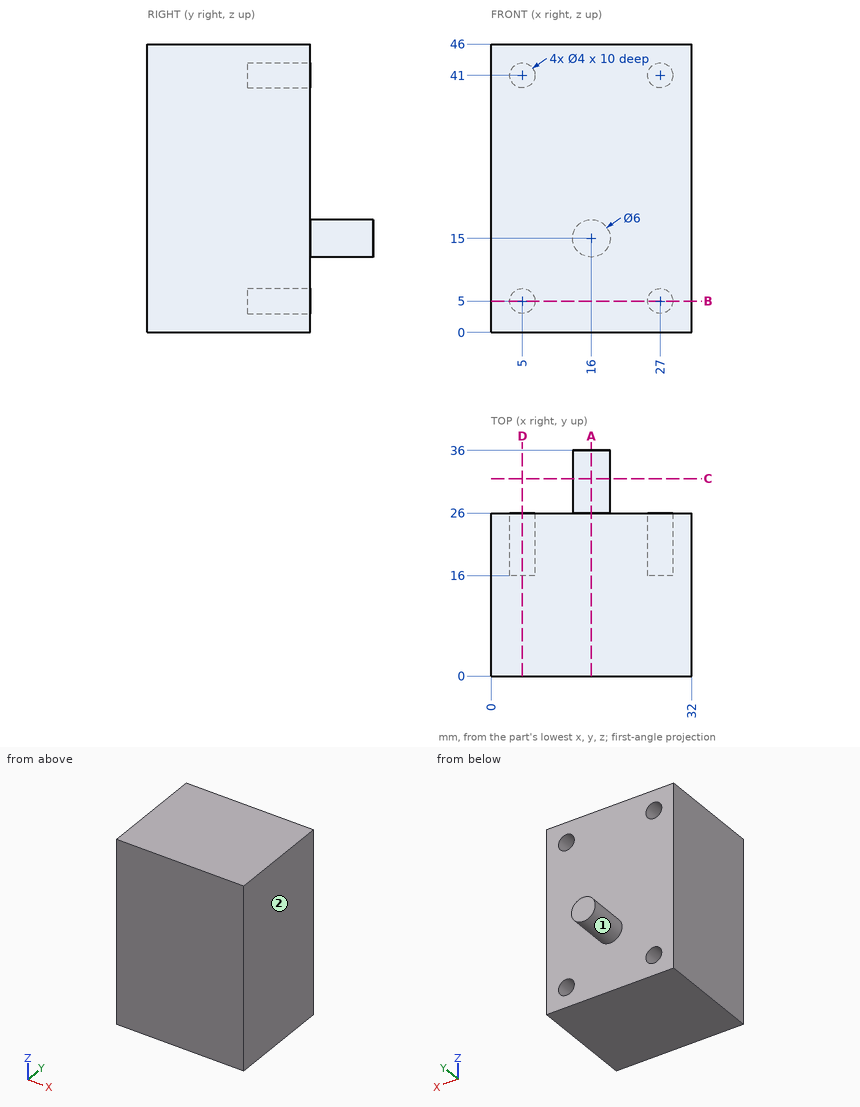
Could you check a few things on this drawing? It's one solid part, dimensions in mm from its lowest x, y, z. A direction names the side the tool comes from. Round coordinates to 2 decimals unless told otherwise and drop trailing zeros. Write each loop counter-clockwise with the first axis right and the second up, starting at its lowest first coordinate (ties: lowest second). Pieces come first, ordered by that corner, then holes. Notation, with made-up numbers: (70, 42) -> (80, 42) arc R19 cw to (80, 46) -> close; hole circle Ø1 at (57.25, 19). An arc over 180 degrees is marked (long way). One line per question, with ' | ' between items. Start each with the question number.
1) I'm going to push flat-ended pins straight in: P1, Ø3, axis at x = 5, z = 41, coming from the +Y side; P2, Ø4.5, axis at x = 27.5, z = 41.5, coming from the +Y side. Where does each tip first touch, or does it pass through?
2) Suppose I cut it at D-D on x = 5. Write out the boundary of the cut face in (y, z), then the cut area to 3 significant figures.
3) Suppose I cut it at A-A on x = 16. Write out the boundary of the cut face in (y, z), then the cut area to 3 significant figures.
4) Suppose I cut it at B-B on z = 5. Write out the boundary of the cut face in (x, y).
5) I need wall thicknesses on line 1 (Z direction, x = 5, y = 20); line 2 (X direction, y = 20, z = 41); line 3 (Z direction, x = 6.5, y = 20). Which ranges of each line are inside material? Lowest first, please. Write a range as [from, to].
6) On a 3-axis mill with a long thin cutter (end or side, diameter ignored), from which of +Z, -Z, +X, -X, +Y, -Y can I reach the whole of each face in a straight line? I mean the marked faces 1 and 2. Say none if no direction works.
7) Suppose I cut it at C-C on y = 31.5. Write out the boundary of the cut face in (x, z), then the cut area to 3 significant figures.
Return value:
1) P1: stops at y = 16 | P2: stops at y = 26
2) outline: (0, 0) -> (26, 0) -> (26, 3) -> (16, 3) -> (16, 7) -> (26, 7) -> (26, 39) -> (16, 39) -> (16, 43) -> (26, 43) -> (26, 46) -> (0, 46) -> close | area: 1,120 mm2
3) outline: (0, 0) -> (26, 0) -> (26, 12) -> (36, 12) -> (36, 18) -> (26, 18) -> (26, 46) -> (0, 46) -> close | area: 1,260 mm2
4) outline: (0, 0) -> (32, 0) -> (32, 26) -> (29, 26) -> (29, 16) -> (25, 16) -> (25, 26) -> (7, 26) -> (7, 16) -> (3, 16) -> (3, 26) -> (0, 26) -> close
5) line 1: z = [0, 3], [7, 39], [43, 46] | line 2: x = [0, 3], [7, 25], [29, 32] | line 3: z = [0, 3.68], [6.32, 39.68], [42.32, 46]
6) face 1: +Y | face 2: +Z, -Z, +X, +Y, -Y
7) outline: circle Ø6 at (16, 15) | area: 28.3 mm2
